Source: CAD feature listing. Evaluate the final solid. Frame: model axes, mm. A direction names the side the tool comes from. Round coordinates to 2 decimals unless told otherwise and drop trailing zeros. Order: outer loops, then holes, each group sorted by start corner. A loop starts at its lowest first (then second) coordinate and runs counter-clockwise, first axis right, second up. Notation, with made-up numbers: (-18.75, -32.5) - (17.25, -32.5) arc R11 cw to (17.25, -19.5) - close; hole circle Ø2 at (17, 64). An arc over 180 degrees is marked (long way). Use one line per item in the form item = value. Start each with the question number.
Q1. Draft query along Z for faces 6 (the cylindrical face through (6.084, -0.924, 6.007)), 7 (the flat face through (20, -52, 0)), 8 (the flat face through (40, -16, 5)). Return one class per face: released by +Z, released by -Z, zero draft, split by the parting line, or undercut.
Q2. Cut plane C-C, the plane x = 20. Give the number of separate pieces and of enclosed holes in the cut face, and give its area (3 significant figures).
Q3. Cut plane A-A, the plane y = 3. Return the cut outline in (x, z), and give its area (3 significant figures).
Q4. Pin query (flat end, axial travel): pin 1 Ø14.5 at (x, y) = (19, -48.5) entering from -Z; pin 2 Ø14.5 at (x, y) = (22.5, 11) entering from +Z; pin 3 Ø10.5 at (x, z) = (23, 28.5) entering from +Y; pin 4 Ø1.5 at (x, y) = (10, -43.5) entering from +Z. Return the tip coordinate at first contact, or that it passes through.
Q5. Set-up query: faces 1 (the flat face through (20, -12.5, 0)), 2 (the flat face through (20, -20, 31)), 3 (the cylindrical face through (19.888, -26.382, -24.172)), 4 (the cylindrical face through (34.084, -0.924, 6.007)), 5 (the cylindrical face through (20, 4, 7)). Return all of +Z, -Z, +X, -X, +Y, -Y with unobstructed straight access to the full face (end or side cutting, diameter ignored); none if empty.
Q6. Ray query, line 1 (Y direction, x = 27, z = -0.5) (3 decimals); line 2 (Y direction, x = 9, z = -0.5); line 3 (X direction, y = 12, z = -9). Return the intervals inside material, ascending. Write a range as [from, to].
Q7. Cut plane B-B, the plane x = 3. Return the cut outline in (y, z), and give its area (3 significant figures).
from build123d import *

# Parameters (mm, degrees)
ESBO_O2_R             = 6
CORTE_EXTRUS_O1_DEPTH = 41
CORTE_EXTRUS_O7_DEPTH = 41
CORTE_EXTRUS_O8_DEPTH = 29
ESBO_O10_R            = 1.3
CORTE_EXTRUS_O9_DEPTH = 41


with BuildPart() as part:
    # Esboço1 → Revolução1 (revolve)
    with BuildSketch(Plane.XY):
        Polygon((0, 0), (12, 0), (12, 18), (28, 18), (28, 0), (40, 0), (40, -20), (0, -20), align=None)
    revolve(axis=Axis((0, -20, 0), (1, 0, 0)))

    # Esboço2 → Corte-extrusão1 (cut, through all)
    with BuildSketch(Plane.ZY):
        with Locations((0, -20)):
            Circle(ESBO_O2_R)
    extrude(amount=-CORTE_EXTRUS_O1_DEPTH, mode=Mode.SUBTRACT)

    # Esboço8 → Corte-extrusão7 (cut, through all)
    with BuildSketch(Plane.ZY):
        Polygon((0, -12.5), (1.5, -12.5), (1.5, -14.653499006), (-1.5, -14.653499006), (-1.5, -12.5), align=None)
    extrude(amount=-CORTE_EXTRUS_O7_DEPTH, mode=Mode.SUBTRACT)

    # Esboço9 → Corte-extrusão8 (cut, through all)
    with BuildSketch(Plane.ZY.offset(-12)):
        with BuildLine():
            Line((0, -58), (0, -45))
            ThreePointArc((0, -45), (-6.470476128, -44.148145657), (-12.5, -41.650635095))
            Line((-12.5, -41.650635095), (-19, -52.908965344))
            ThreePointArc((-19, -52.908965344), (-9.835123714, -56.705181399), (0, -58))
        make_face()
        with BuildLine():
            Line((19, 12.908965344), (12.5, 1.650635095))
            ThreePointArc((12.5, 1.650635095), (6.470476128, 4.148145657), (0, 5))
            Line((0, 5), (0, 18))
            ThreePointArc((0, 18), (9.835123714, 16.705181399), (19, 12.908965344))
        make_face()
        with BuildLine():
            Line((-19, 12.908965344), (-12.5, 1.650635095))
            ThreePointArc((-12.5, 1.650635095), (-17.67766953, -2.32233047), (-21.650635095, -7.5))
            Line((-21.650635095, -7.5), (-32.908965344, -1))
            ThreePointArc((-32.908965344, -1), (-26.870057685, 6.870057685), (-19, 12.908965344))
        make_face()
        with BuildLine():
            Line((32.908965344, -1), (21.650635095, -7.5))
            ThreePointArc((21.650635095, -7.5), (24.148145657, -13.529523872), (25, -20))
            Line((25, -20), (38, -20))
            ThreePointArc((38, -20), (36.705181399, -10.164876286), (32.908965344, -1))
        make_face()
        with BuildLine():
            Line((19, -52.908965344), (12.5, -41.650635095))
            ThreePointArc((12.5, -41.650635095), (17.67766953, -37.67766953), (21.650635095, -32.5))
            Line((21.650635095, -32.5), (32.908965344, -39))
            ThreePointArc((32.908965344, -39), (26.870057685, -46.870057685), (19, -52.908965344))
        make_face()
        with BuildLine():
            Line((-38, -20), (-25, -20))
            ThreePointArc((-25, -20), (-24.148145657, -26.470476128), (-21.650635095, -32.5))
            Line((-21.650635095, -32.5), (-32.908965344, -39))
            ThreePointArc((-32.908965344, -39), (-36.705181399, -29.835123714), (-38, -20))
        make_face()
    extrude(amount=-CORTE_EXTRUS_O8_DEPTH, mode=Mode.SUBTRACT)

    # Esboço10 → Corte-extrusão9 (cut, through all)
    with BuildSketch(Plane.ZY):
        with Locations((0, -5.003986953)):
            Circle(ESBO_O10_R)
        with Locations((14.996013047, -20)):
            Circle(ESBO_O10_R)
        with Locations((0, -34.996013047)):
            Circle(ESBO_O10_R)
        with Locations((-14.996013047, -20)):
            Circle(ESBO_O10_R)
    extrude(amount=-CORTE_EXTRUS_O9_DEPTH, mode=Mode.SUBTRACT)


solid = part.part
Completed:
q1.face_6 = split by the parting line
q1.face_7 = undercut
q1.face_8 = zero draft
q2.separate_pieces = 1
q2.enclosed_holes = 5
q2.area = 3,110 mm2
q3.outline = (12, -13.28) - (28, -13.28) - (28, 9.8) - (12, 9.8) - close; (12, 13.28) - (28, 13.28) - (28, 30.25) - (12, 30.25) - close
q3.area = 641 mm2
q4.pin_1 = -31.5
q4.pin_2 = 29.66
q4.pin_3 = 10.06
q4.pin_4 = through
q5.face_1 = +X, -X
q5.face_2 = +Z, +X, -X
q5.face_3 = -Z, +X, -X
q5.face_4 = +X
q5.face_5 = +X, -X, +Y
q6.line_1 = [-44.995, -36.196], [-33.796, -25.979], [-12.5, -6.204], [-3.804, 17.997]
q6.line_2 = [-39.99, -36.2], [-33.8, -25.98], [-12.5, -6.2], [-3.8, -0.01]
q6.line_3 = [12, 28]
q7.outline = circle Ø40 at (-20, 0); hole circle Ø2.6 at (-35, 0); hole circle Ø2.6 at (-20, -15); hole circle Ø2.6 at (-20, 15); hole (-14.19, -1.5) - (-12.5, -1.5) - (-12.5, 1.5) - (-14.19, 1.5) arc R6 ccw (long way) to start; hole circle Ø2.6 at (-5, 0)
q7.area = 1,120 mm2
